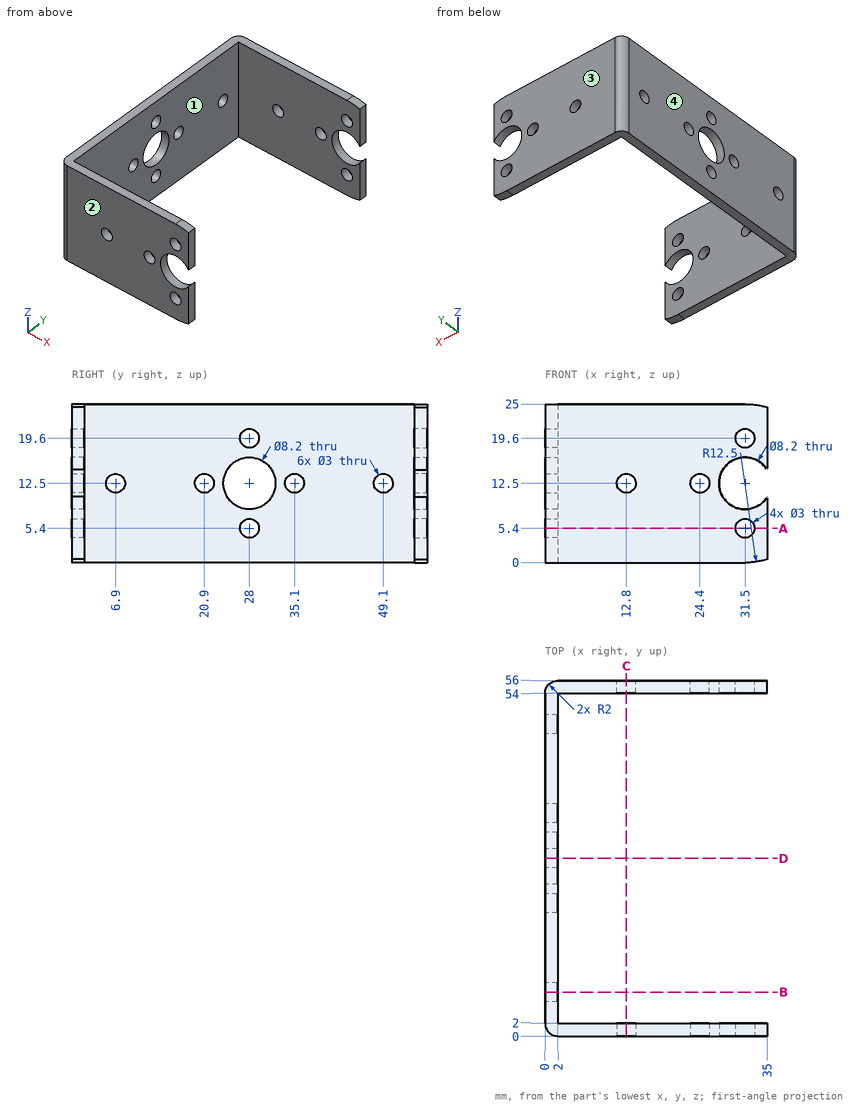
Here's the drawing with two shaded views (mm, measured from the low corner). I have some questions. Give positions to 0.01 mm unless a question says otherwise; leave off trailing zeros. Loops run counter-clockwise (first coordinate to the right, second up) from the corner with the lowest first, then second, coordinate; pieces in that order, holes last. Notation, with made-up numbers: M 2,47 L 44,47 A10 cw 44,64 Z; hole C 23.25,9.25 d10. An arc over 180 degrees is marked long. Answer in a Markdown table with one row per item.
1. Suppose I cut it at B-B on y = 6.9. Write out the boundary of the cut face in (x, z), plus the area to 3 significant figures.
Taken from the geometry:
| item | result |
|---|---|
| outline | M 0,0 L 2,0 L 2,11 L 0,11 Z; M 0,14 L 2,14 L 2,25 L 0,25 Z |
| area | 44.0 mm² |
2. If I drill on line 1 along Y through (x, z) = (28.5, 7); line 2 along X through (y, z) = (55.25, 12.5); line 3 along X through (y, z) = (52.5, 5), over which ranges is the centre line in solid material (lowest first)?
Taken from the geometry:
| item | result |
|---|---|
| line 1 | y = 0 to 2, 54 to 56 |
| line 2 | x = 0.44 to 11.3, 14.3 to 22.9, 25.9 to 27.4 |
| line 3 | x = 0 to 2 |
3. Suppose I cut it at C-C on x = 12.8. Write out the boundary of the cut face in (y, z).
Taken from the geometry:
| item | result |
|---|---|
| outline | M 0,0 L 2,0 L 2,11 L 0,11 Z; M 0,14 L 2,14 L 2,25 L 0,25 Z; M 54,0 L 56,0 L 56,11 L 54,11 Z; M 54,14 L 56,14 L 56,25 L 54,25 Z |
4. Suppose I cut it at A-A on z = 5.4. Write out the boundary of the cut face in (x, y).
Taken from the geometry:
| item | result |
|---|---|
| outline | M 0,2 A2 ccw 2,0 L 30,0 L 30,2 L 2,2 L 2,26.5 L 0,26.5 Z; M 0,29.5 L 2,29.5 L 2,54 L 30,54 L 30,56 L 2,56 A2 ccw 0,54 Z; M 33,0 L 35,0 L 35,2 L 33,2 Z; M 33,54 L 35,54 L 35,56 L 33,56 Z |
5. Suppose I cut it at D-D on y = 28. Write out the boundary of the cut face in (x, z), plus the area to 3 significant figures.
Taken from the geometry:
| item | result |
|---|---|
| outline | M 0,0 L 2,0 L 2,3.9 L 0,3.9 Z; M 0,6.9 L 2,6.9 L 2,8.4 L 0,8.4 Z; M 0,16.6 L 2,16.6 L 2,18.1 L 0,18.1 Z; M 0,21.1 L 2,21.1 L 2,25 L 0,25 Z |
| area | 21.6 mm² |
6. For pin 1 Ø5 at (y, z) = (34, 9.5) entering from +X, with a flat end and sliding along its axis, tell me the tip position at first contact or that it passes through.
Taken from the geometry:
| item | result |
|---|---|
| pin 1 | stops at x = 2 |
7. Thinking about a two-plate mould opening in Y: for the marked faces 1, 2, 3 and 4, which applies, released by +Y, released by -Y, zero draft, split by the parting line, or undercut?
Taken from the geometry:
| item | result |
|---|---|
| face 1 | undercut |
| face 2 | released by -Y |
| face 3 | released by +Y |
| face 4 | zero draft |
